The figure shows three views and two pictorial views of one solid part (mm, origin at its lowest corner). Answer the questions. A direction names the side the tool comes from. Coordinates: 2 decimals unless noted, no trailing zeros. Write each loop counter-clockwise with the first axis right and the second up, starting at its lowest first coordinate (ties: lowest second). Pieces come first, ordered by that corner, then holes.
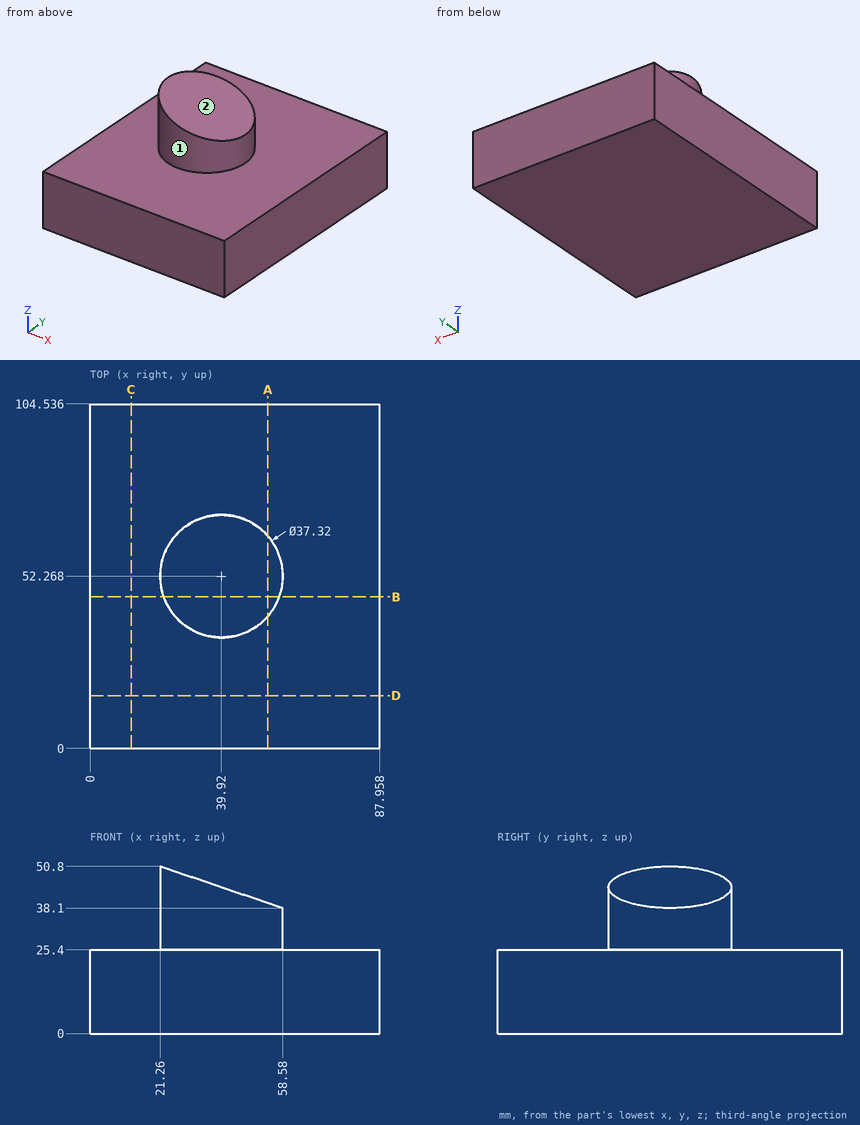
1. Section B-B on y = 46 is taken. Give the vertices of the cut face in (x, z) (1 decimal).
Results found:
outline: (0, 0) - (88, 0) - (88, 25.4) - (57.5, 25.4) - (57.5, 38.5) - (22.3, 50.4) - (22.3, 25.4) - (0, 25.4) - close
2. Flat-ended cylindrical pins translate along their axes: P1, Ø3, axis at x = 27, z = 36.5, coming from the -Y side; P2, Ø4, axis at x = 71, y = 90.5, coming from the +Z side; P3, Ø3, axis at x = 54, z = 41.5, coming from the -Y side; P4, Ø1.5, axis at y = 35.5, z = 35, coming from the +X side. Find the tip coordinate at first contact, or state that the pin passes through.
Results found:
P1: stops at y = 37.51
P2: stops at z = 25.4
P3: passes through
P4: stops at x = 49.49
3. Find the intervals of material crossed by L1, parallel to Z at x = 65, y = 16; L2, parallel to Z at x = 34.5, y = 38.5 (1 decimal); L3, parallel to Y at x = 46.5, z = 36, in increasing order.
Results found:
L1: z = 0 to 25.4
L2: z = 0 to 46.3
L3: y = 34.81 to 69.73
4. Section D-D on y = 16 is taken. Give the vertices of the cut face in (x, z).
Results found:
outline: (0, 0) - (87.96, 0) - (87.96, 25.4) - (0, 25.4) - close
5. Section C-C on x = 12.5 is taken. Give the vertices of the cut face in (y, z).
Results found:
outline: (0, 0) - (104.54, 0) - (104.54, 25.4) - (0, 25.4) - close
6. Section A-A on x = 54 is taken. Give the vertices of the cut face in (y, z).
Results found:
outline: (0, 0) - (104.54, 0) - (104.54, 25.4) - (64.51, 25.4) - (64.51, 39.66) - (40.02, 39.66) - (40.02, 25.4) - (0, 25.4) - close
7. A tool of negligible diameter and unlimited length cuts with its end or side. For the marked faces 1 and 2, from which of +Z, -Z, +X, -X, +Y, -Y can it reach the whole face along a straight path? Write none if from no direction.
Results found:
face 1: +Z
face 2: +Z, +X, +Y, -Y
